For this review, take the finished solid that the model builds, in its own axes (mm). A direction names the side the tool comes from. Round coordinates to 2 decimals unless told otherwise and drop trailing zeros. Write each loop counter-clockwise with the first axis right and the second up, starting at its lowest first coordinate (ties: lowest second). Pieces come first, ordered by that corner, then holes. Notation, with made-up numbers: M -8.75,56 L 45.25,56 A35 cw 45.25,89 Z; hole C -21.5,62.5 d6. An arc over 180 degrees is marked long. Answer in a Markdown table with one row per item.
```python
from build123d import *

# Parameters (mm, degrees)
BOSS_EXTRUDE1_DEPTH  = 100
MIRROR3_COPY_1_DEPTH = 100
MIRROR3_COPY_2_DEPTH = 100


with BuildPart() as part:
    # Sketch1 → Boss-Extrude1 (new body)
    with BuildSketch(Plane.XY):
        with BuildLine():
            Line((3.4, 0), (5.5, 0))
            Line((5.5, 0), (5.5, 4))
            Line((5.5, 4), (11.69, 10.19))
            Line((11.69, 10.19), (18.2, 10.19))
            Line((18.2, 10.19), (18.2, 5.265595036))
            Line((18.2, 5.265595036), (15.5, 5.265595036))
            Line((15.5, 5.265595036), (15.5, 2.965595036))
            Line((15.5, 2.965595036), (19, 2.965595036))
            Line((19, 2.965595036), (19, 3.965595036))
            Line((19, 3.965595036), (20, 3.965595036))
            Line((20, 3.965595036), (20, 15.5))
            ThreePointArc((20, 15.5), (18.681980515, 18.681980515), (15.5, 20))
            Line((15.5, 20), (6.385304712, 20))
            Line((6.385304712, 20), (6.385304712, 19))
            Line((6.385304712, 19), (5.385304712, 19))
            Line((5.385304712, 19), (5.385304712, 15.5))
            Line((5.385304712, 15.5), (7.685304712, 15.5))
            Line((7.685304712, 15.5), (7.685304712, 18.2))
            Line((7.685304712, 18.2), (10.19, 18.2))
            Line((10.19, 18.2), (10.19, 11.69))
            Line((10.19, 11.69), (4, 5.5))
            Line((4, 5.5), (0, 5.5))
            Line((0, 5.5), (0, 3.4))
            ThreePointArc((0, 3.4), (2.404163056, 2.404163056), (3.4, 0))
        make_face()
        with BuildLine():
            Line((18.5, 11.69), (18.5, 15.5))
            ThreePointArc((18.5, 15.5), (17.621320344, 17.621320344), (15.5, 18.5))
            Line((15.5, 18.5), (11.69, 18.5))
            Line((11.69, 18.5), (11.69, 11.69))
            Line((11.69, 11.69), (18.5, 11.69))
        make_face(mode=Mode.SUBTRACT)
    boss_extrude1 = extrude(amount=BOSS_EXTRUDE1_DEPTH)

    # Mirror1: Boss-Extrude1 across plane
    add(boss_extrude1.mirror(Plane.ZX))

    # Mirror2: Boss-Extrude1 across plane
    add(boss_extrude1.mirror(Plane(origin=(0, 0, 0), x_dir=(0, 0, 1), z_dir=(1, 0, 0))))

    # Mirror3 copy 1 sketch → Mirror3 copy 1 (add)
    with BuildSketch(Plane(origin=(0, 0, 0), x_dir=(-1, 0, 0), z_dir=(0, 0, 1))):
        with BuildLine():
            Line((3.4, 0), (5.5, 0))
            Line((5.5, 0), (5.5, 4))
            Line((5.5, 4), (11.69, 10.19))
            Line((11.69, 10.19), (18.2, 10.19))
            Line((18.2, 10.19), (18.2, 5.265595036))
            Line((18.2, 5.265595036), (15.5, 5.265595036))
            Line((15.5, 5.265595036), (15.5, 2.965595036))
            Line((15.5, 2.965595036), (19, 2.965595036))
            Line((19, 2.965595036), (19, 3.965595036))
            Line((19, 3.965595036), (20, 3.965595036))
            Line((20, 3.965595036), (20, 15.5))
            ThreePointArc((20, 15.5), (18.681980515, 18.681980515), (15.5, 20))
            Line((15.5, 20), (6.385304712, 20))
            Line((6.385304712, 20), (6.385304712, 19))
            Line((6.385304712, 19), (5.385304712, 19))
            Line((5.385304712, 19), (5.385304712, 15.5))
            Line((5.385304712, 15.5), (7.685304712, 15.5))
            Line((7.685304712, 15.5), (7.685304712, 18.2))
            Line((7.685304712, 18.2), (10.19, 18.2))
            Line((10.19, 18.2), (10.19, 11.69))
            Line((10.19, 11.69), (4, 5.5))
            Line((4, 5.5), (0, 5.5))
            Line((0, 5.5), (0, 3.4))
            ThreePointArc((0, 3.4), (2.404163056, 2.404163056), (3.4, 0))
        make_face()
        with BuildLine():
            Line((18.5, 11.69), (18.5, 15.5))
            ThreePointArc((18.5, 15.5), (17.621320344, 17.621320344), (15.5, 18.5))
            Line((15.5, 18.5), (11.69, 18.5))
            Line((11.69, 18.5), (11.69, 11.69))
            Line((11.69, 11.69), (18.5, 11.69))
        make_face(mode=Mode.SUBTRACT)
    extrude(amount=MIRROR3_COPY_1_DEPTH)

    # Mirror3 copy 2 sketch → Mirror3 copy 2 (add)
    with BuildSketch(Plane.XY):
        with BuildLine():
            Line((3.4, 0), (5.5, 0))
            Line((5.5, 0), (5.5, -4))
            Line((5.5, -4), (11.69, -10.19))
            Line((11.69, -10.19), (18.2, -10.19))
            Line((18.2, -10.19), (18.2, -5.265595036))
            Line((18.2, -5.265595036), (15.5, -5.265595036))
            Line((15.5, -5.265595036), (15.5, -2.965595036))
            Line((15.5, -2.965595036), (19, -2.965595036))
            Line((19, -2.965595036), (19, -3.965595036))
            Line((19, -3.965595036), (20, -3.965595036))
            Line((20, -3.965595036), (20, -15.5))
            ThreePointArc((20, -15.5), (18.681980515, -18.681980515), (15.5, -20))
            Line((15.5, -20), (6.385304712, -20))
            Line((6.385304712, -20), (6.385304712, -19))
            Line((6.385304712, -19), (5.385304712, -19))
            Line((5.385304712, -19), (5.385304712, -15.5))
            Line((5.385304712, -15.5), (7.685304712, -15.5))
            Line((7.685304712, -15.5), (7.685304712, -18.2))
            Line((7.685304712, -18.2), (10.19, -18.2))
            Line((10.19, -18.2), (10.19, -11.69))
            Line((10.19, -11.69), (4, -5.5))
            Line((4, -5.5), (0, -5.5))
            Line((0, -5.5), (0, -3.4))
            ThreePointArc((0, -3.4), (2.404163056, -2.404163056), (3.4, 0))
        make_face()
        with BuildLine():
            Line((18.5, -11.69), (18.5, -15.5))
            ThreePointArc((18.5, -15.5), (17.621320344, -17.621320344), (15.5, -18.5))
            Line((15.5, -18.5), (11.69, -18.5))
            Line((11.69, -18.5), (11.69, -11.69))
            Line((11.69, -11.69), (18.5, -11.69))
        make_face(mode=Mode.SUBTRACT)
    extrude(amount=MIRROR3_COPY_2_DEPTH)


solid = part.part
```
Q1. Take a section at C-C (y = 1). State the section outline as (x, z) points, then the cut area to 3 significant figures.
Found:
| item | result |
|---|---|
| outline | M -5.5,0 L -3.25,0 L -3.25,100 L -5.5,100 Z; M 3.25,0 L 5.5,0 L 5.5,100 L 3.25,100 Z |
| area | 450 mm² |
Q2. Take a section at D-D (z = 10). State how many separate pieces and enclosed holes the cut face has, then the cut area to 3 significant figures.
Found:
| item | result |
|---|---|
| separate pieces | 1 |
| enclosed holes | 5 |
| area | 468 mm² |
Q3. Machinability: for faces 5 (the face through (-5.385, 17, 49)), 6 (the face through (18.717, -18.647, 49.3)), 7 (the face through (17, 2.966, 49)), 8 (the face through (3, -2, 0)), 9 (the face through (15, 10.19, 49)), which of the approach directions +Z, -Z, +X, -X, +Y, -Y give a long, thin tool a straight path to every point of the face, cutting with its end or side? Answer none if there is none.
Found:
| item | result |
|---|---|
| face 5 | +Z, -Z, +Y |
| face 6 | +Z, -Z, +X, -Y |
| face 7 | +Z, -Z, +X |
| face 8 | -Z, +X, -X, +Y, -Y |
| face 9 | +Z, -Z |
Q4. Take a section at A-A (y = 8). State the section outline as (x, z) points.
Found:
| item | result |
|---|---|
| outline | M -20,0 L -18.2,0 L -18.2,100 L -20,100 Z; M -9.5,0 L -6.5,0 L -6.5,100 L -9.5,100 Z; M 6.5,0 L 9.5,0 L 9.5,100 L 6.5,100 Z; M 18.2,0 L 20,0 L 20,100 L 18.2,100 Z |
Q5. Insertion check: P1, Ø1.1, axis at y = -19.5, z = 37, coming from the -X side; P2, Ø8, axis at x = -4, z = 85, coming from the -Y side; P3, Ø3, axis at y = 0, z = 38, coming from the +X side; P4, Ø1.8, axis at y = -17.5, z = 65, coming from the +X side. Each pin has a flat end and moves straight along its axis. Give the tip position at first contact, or say it passes through.
Found:
| item | result |
|---|---|
| P1 | x = -18.39 |
| P2 | y = -20 |
| P3 | x = 5.5 |
| P4 | x = 19.86 |
Q6. Mouldability with a two-part tool opening along X and no side actions: class faces 1 (the face through (15, -11.69, 49)), 2 (the face through (17, -2.966, 49)), 3 (the face through (20, 10, 49)), 4 (the face through (-15, -11.69, 49)) as +X half, -X half, draft (parallel to the pull), parting line (faces both ways), or undercut.
Found:
| item | result |
|---|---|
| face 1 | undercut |
| face 2 | draft |
| face 3 | +X half |
| face 4 | undercut |
Q7. For probe 1 along Y at (x, z) = (-12.5, 29); probe 2 along X at (y, z) = (-3.5, 66); probe 3 along X at (y, z) = (-16, 51.5), list the stretches that pass through material, from the lowest coordinate up.
Found:
| item | result |
|---|---|
| probe 1 | -20 to -18.5, -11.69 to -10.19, 10.19 to 11.69, 18.5 to 20 |
| probe 2 | -19 to -15.5, -5.5 to 5.5, 15.5 to 19 |
| probe 3 | -19.97 to -18.46, -11.69 to -10.19, -7.69 to -5.39, 5.39 to 7.69, 10.19 to 11.69, 18.46 to 19.97 |
Q8. Take a section at B-B (x = -13.5). State the section outline as (y, z) points.
Found:
| item | result |
|---|---|
| outline | M -20,0 L -18.5,0 L -18.5,100 L -20,100 Z; M -11.69,0 L -10.19,0 L -10.19,100 L -11.69,100 Z; M 10.19,0 L 11.69,0 L 11.69,100 L 10.19,100 Z; M 18.5,0 L 20,0 L 20,100 L 18.5,100 Z |
